from build123d import *

# Parameters (mm, degrees)
SKETCH1_W             = 75
SKETCH1_H             = 35
BOSS_EXTRUDE1_DEPTH   = 12
CUT_EXTRUDE1_REACH    = 45.087
M8X1_0_TAPPED_HOLE1_D = 7
CHAMFER1_SIZE         = 2


with BuildPart() as part:
    # Sketch1 → Boss-Extrude1 (new body)
    with BuildSketch(Plane.XY):
        Rectangle(SKETCH1_W, SKETCH1_H)
    extrude(amount=BOSS_EXTRUDE1_DEPTH)

    # Sketch2 → Cut-Extrude1 (cut, up to next)
    with BuildSketch(Plane(origin=(0, 0, 0), x_dir=(-1, 0, 0), z_dir=(0, 0, -1)), mode=Mode.PRIVATE) as cut_extrude1_sk1:
        with BuildLine():
            Line((-8.73125, 0), (-8.73125, -17.5))
            Line((-8.73125, -17.5), (8.73125, -17.5))
            Line((8.73125, -17.5), (8.73125, 0))
            ThreePointArc((8.73125, 0), (0, 8.73125), (-8.73125, 0))
        make_face()
    cut_extrude1_tool1 = extrude(cut_extrude1_sk1.sketch, amount=-CUT_EXTRUDE1_REACH, mode=Mode.PRIVATE) & part.part
    add(cut_extrude1_tool1.solids().sort_by_distance((0, -5.243288, 0))[0], mode=Mode.SUBTRACT)

    # M8x1.0 Tapped Hole1 (through all)
    with Locations(Plane.XY.offset(12)):
        with Locations((-25.5, 0), (25.5, 0)):
            Hole(M8X1_0_TAPPED_HOLE1_D / 2)

    # Chamfer1
    chamfer1_edges = [part.edges().sort_by_distance(p)[0] for p in [
        (-8.73125, -17.5, 6),
        (8.73125, -17.5, 6),
    ]]
    chamfer(chamfer1_edges, length=CHAMFER1_SIZE)


solid = part.part
Input: part model. Units: mm. Frame: model coordinates. A direction names the side the tool comes from. Coordinates: 2 decimals unless noted, no trailing zeros. Write each loop counter-clockwise with the first axis right and the second up, starting at its lowest first coordinate (ties: lowest second). Pieces come first, ordered by that corner, then holes. Notation, with made-up numbers: M -23,53 L 30,53 A27 cw 30,90 Z; hole C 77,87.25 d8. An arc over 180 degrees is marked long. Answer as a JSON object with one key per item and string values. Group by question number.
(1) Section B-B on x = 25.5. Output: boundary loops of the cut face in (y, z).
(2) Section D-D on y = -2. Output: boundary loops of the cut face in (x, z).
(3) Set-up query: faces 5 (the face through (24, -17.5, 6)), 6 (the face through (-8.731, -8, 6)). Return all of +Z, -Z, +X, -X, +Y, -Y with unobstructed straight access to the full face (end or side cutting, diameter ignored); none if empty.
(4) Section A-A on y = -14.5. Output: boundary loops of the cut face in (x, z).
(5) Mould query, pull axis X, two halves, no side actions, for faces 1 (the face through (22.16, 1.05, 5.92)), 2 (the face through (-37.5, 0, 6)), 3 (the face through (-28.84, 1.05, 5.92)), 4 (the face through (-9, 0, 12)). Classes: pulls with the +X half, pulls with the -X half, needs draft (parallel to the pull), parting line crosses it, or undercut.
(6) Section C-C on z = 11.25. Output: boundary loops of the cut face in (x, y).
(7) Ray query, line 1 along X through (y, z) = (-2, 9.25); line 2 along Y through (x, z) = (25.5, 6.5); line 3 along X through (y, z) = (-8, 4.5). Return the intervals inside material, ascending. Write a range as [from, to].
Result set:
{
 "1": {"outline": "M -17.5,0 L -3.5,0 L -3.5,12 L -17.5,12 Z; M 3.5,0 L 17.5,0 L 17.5,12 L 3.5,12 Z"},
 "2": {"outline": "M -37.5,0 L -28.37,0 L -28.37,12 L -37.5,12 Z; M -22.63,0 L -8.73,0 L -8.73,12 L -22.63,12 Z; M 8.73,0 L 22.63,0 L 22.63,12 L 8.73,12 Z; M 28.37,0 L 37.5,0 L 37.5,12 L 28.37,12 Z"},
 "3": {"face 5": "+Z, -Z, +X, -X, -Y", "face 6": "+Z, -Z, -Y"},
 "4": {"outline": "M -37.5,0 L -8.73,0 L -8.73,12 L -37.5,12 Z; M 8.73,0 L 37.5,0 L 37.5,12 L 8.73,12 Z"},
 "5": {"face 1": "undercut", "face 2": "pulls with the -X half", "face 3": "undercut", "face 4": "needs draft"},
 "6": {"outline": "M -37.5,-17.5 L -10.73,-17.5 L -8.73,-15.5 L -8.73,0 A8.73 cw 8.73,0 L 8.73,-15.5 L 10.73,-17.5 L 37.5,-17.5 L 37.5,17.5 L -37.5,17.5 Z; hole C -25.5,0 d7; hole C 25.5,0 d7"},
 "7": {"line 1": "x = [-37.5, -28.37], [-22.63, -8.73], [8.73, 22.63], [28.37, 37.5]", "line 2": "y = [-17.5, -3.5], [3.5, 17.5]", "line 3": "x = [-37.5, -8.73], [8.73, 37.5]"}
}
